CAD build for the part. Positions are in the model's coordinates, mm. A direction names the side the tool comes from. Give positions to 0.01 mm unless a question says otherwise; leave off trailing zeros. Loops run counter-clockwise (first coordinate to the right, second up) from the corner with the lowest first, then second, coordinate; pieces in that order, holes last.
```python
from build123d import *

# Parameters (mm, degrees)
SKETCH1_W              = 31.75
SKETCH1_H              = 31.75
BOSS_EXTRUDE1_DEPTH    = 50.8
CUT_EXTRUDE1_DEPTH     = 68.7994469
SKETCH3_W              = 12.7
SKETCH3_H              = 50.8
CUT_EXTRUDE2_DEPTH     = 63.206798736
F_1_1_DIAMETER_HOLE1_D = 6.35
F_1_1_DIAMETER_HOLE2_D = 6.35


with BuildPart() as part:
    # Sketch1 → Boss-Extrude1 (new body)
    with BuildSketch(Plane(origin=(0, 0, 0), x_dir=(1, 0, 0), z_dir=(0, 1, 0))):
        with Locations((15.875, 15.875)):
            Rectangle(SKETCH1_W, SKETCH1_H)
    extrude(amount=BOSS_EXTRUDE1_DEPTH)

    # Sketch2 → Cut-Extrude1 (cut, through all)
    with BuildSketch(Plane(origin=(31.75, 0, 0), x_dir=(0, 0, -1), z_dir=(1, 0, 0))):
        with BuildLine():
            Line((0, 50.8), (31.75, 50.8))
            Line((31.75, 50.8), (31.75, 27.178))
            ThreePointArc((31.75, 27.178), (15.875, 43.053), (0, 27.178))
            Line((0, 27.178), (0, 50.8))
        make_face()
    extrude(amount=-CUT_EXTRUDE1_DEPTH, mode=Mode.SUBTRACT)

    # Sketch3 → Cut-Extrude2 (cut, through all)
    with BuildSketch(Plane.XY):
        with Locations((15.875, 31.75)):
            Rectangle(SKETCH3_W, SKETCH3_H)
    extrude(amount=-CUT_EXTRUDE2_DEPTH, mode=Mode.SUBTRACT)

    # 1 (1) Diameter Hole1 (through all)
    with Locations(Plane(origin=(0, 6.35, 0), x_dir=(1, 0, 0), z_dir=(0, 1, 0))):
        with Locations((15.875, 23.8125), (15.875, 7.9375)):
            Hole(F_1_1_DIAMETER_HOLE1_D / 2)

    # 1 (1) Diameter Hole2 (through all)
    with Locations(Plane(origin=(31.75, 0, 0), x_dir=(0, 0, -1), z_dir=(1, 0, 0))):
        with Locations((15.875, 27.178)):
            Hole(F_1_1_DIAMETER_HOLE2_D / 2)


solid = part.part
```
1. Saw through at D-D, the plane x = 3. List the corners of the cut face in (y, z) (3 decimals), and give its area (3 significant figures).
Responses:
outline: (0, -31.75) - (27.178, -31.75) arc R15.875 ccw to (27.178, 0) - (0, 0) - close; hole circle Ø6.35 at (27.178, -15.875)
area: 1,230 mm2
2. Pull direction Y, two halves, no side cores. Call faces 3 (the face through (4.83, 43.05, -16.22)), 4 (the face through (14.41, 3.13, -5.12)), 5 (the face through (26.921, 25.962, -12.942)): released by +Y, released by -Y, zero draft, split by the parting line, or undercut.
Responses:
face 3: released by +Y
face 4: zero draft
face 5: undercut
3. Saw through at B-B, the plane z = -18. List the corners of the cut face in (x, y) (3 decimals).
Responses:
outline: (0, 0) - (31.75, 0) - (31.75, 24.819) - (22.225, 24.819) - (22.225, 6.35) - (9.525, 6.35) - (9.525, 24.819) - (0, 24.819) - close; (0, 29.537) - (9.525, 29.537) - (9.525, 42.91) - (0, 42.91) - close; (22.225, 29.537) - (31.75, 29.537) - (31.75, 42.91) - (22.225, 42.91) - close
4. Saw through at C-C, the plane z = -26. List the corners of the cut face in (x, y) (3 decimals), and give its area (3 significant figures).
Responses:
outline: (0, 0) - (13.574, 0) - (13.574, 6.35) - (9.525, 6.35) - (9.525, 39.405) - (0, 39.405) - close; (18.176, 0) - (31.75, 0) - (31.75, 39.405) - (22.225, 39.405) - (22.225, 6.35) - (18.176, 6.35) - close
area: 802 mm2
5. Drop flat-ended pins along their axis: pin 1 (10 mm diameter, centred on x = 15.88, z = -7.94, fed in from +Y); pin 2 (5.5 mm diameter, centred on y = 27.178, z = -15.875, fed in from -X); pin 3 (3 mm diameter, centred on x = 4.5, z = -24.5, fed in from +Y); pin 4 (1 mm diameter, centred on x = 23, y = 30.5, fed in from -Z). Give the stop position or say it passes through.
Responses:
pin 1: stops at y = 6.35
pin 2: passes through
pin 3: stops at y = 41.36
pin 4: stops at z = -31.5
6. Probe line 1 along X through (y, z) = (16, -22) (3 decimals); line 2 along Z through (x, y) = (13, 5.5); line 3 along Y through (x, z) = (10, -16). List the from-to ranges inside material, lowest first.
Responses:
line 1: x = 0 to 9.525, 22.225 to 31.75
line 2: z = -31.75 to -25.16, -22.47 to -9.28, -6.59 to 0
line 3: y = 0 to 6.35
7. Tool access for faces 1 (the face through (22.225, 20, -16)), 2 (the face through (14.4, 3.1, -21)): list every direction of +Z, -Z, +X, -X, +Y, -Y with a clear straight run to the whole face (end or side of a thin tool).
Responses:
face 1: +Z, -Z, +Y
face 2: +Y, -Y
8. Saw through at A-A, the plane y = 12.5. List the corners of the cut face in (x, z) (3 decimals).
Responses:
outline: (0, -31.75) - (9.525, -31.75) - (9.525, 0) - (0, 0) - close; (22.225, -31.75) - (31.75, -31.75) - (31.75, 0) - (22.225, 0) - close
